Check sheet for the modelled part. Datum: model origin and axes. Units: mm. A direction names the side the tool comes from. Round coordinates to 2 decimals unless told otherwise and drop trailing zeros. Loops run counter-clockwise (first coordinate to the right, second up) from the corner with the lowest first, then second, coordinate; pieces in that order, holes last. Notation, with made-up numbers: M 38,68.5 L 80,68.5 A16 ccw 80,93.5 Z; hole C -9,-35 d3. An arc over 180 degrees is marked long. Write item = value, one per line. Start each with the question number.
(1) Scan lines: L1, parallel to Y at x = -0.05, z = 0.9; L2, parallel to X at y = 20, z = 1.6; L3, parallel to Y at x = -0.1, z = 0.45. Record each from-to range of solid material in increasing order. Write a range as from..to.
(2) Mould release check, pull along Y, two halves, no side actions. Record for faces 3 (the face through (-0.325, 21.464, 1.479)), 4 (the face through (1, 0, 0)): pulls with the +Y half, pulls with the -Y half, needs draft (parallel to the pull), parting line crosses it, or undercut.
(3) Cross-section at B-B on z = 0.25. Record the boundary of the cut face in (x, y).
(4) Cross-section at D-D on z = 1.9. Record the boundary of the cut face in (x, y).
(5) Cross-section at A-A on y = 20. Record the boundary of the cut face in (x, z).
(6) Cross-section at C-C on x = -0.2. Record the boundary of the cut face in (y, z), plus the area to 3 significant figures.
(7) Go/stop test with a flat-tipped pin: P1, Ø1, axis at y = 18, z = 2.5, coming from the -X side. Record where the tip stops, or that it passes through.
(8) Set-up check for faces 1 (the face through (-0.976, 9.876, 1.283)), 2 (the face through (-0.108, -0.488, 1.479)): record each of +Z, -Z, +X, -X, +Y, -Y from which the full face is reachable in a straight line by a thin tool's end or side.
from build123d import *

# Parameters (mm, degrees)
SKETCH_1_R           = 1.5
SKETCH_1_R_2         = 0.5
EXTRUDE_1_DEPTH      = 3
EXTRUDE_2_REACH      = 13.979
EXTRUDE_2_END_RADIUS = 1.5
SKETCH_2_R           = 1


with BuildPart() as part:
    # 草图1 → 凸台-拉伸1 (new body)
    with BuildSketch(Plane.XY):
        Circle(SKETCH_1_R)
        Circle(SKETCH_1_R_2, mode=Mode.SUBTRACT)
    extrude_1 = extrude(amount=EXTRUDE_1_DEPTH)

    # 凸台-拉伸2: up to this cylinder (the profile starts outside it)
    extrude_2_end = Plane(origin=(0, 0, 1.5), z_dir=(0, 0, -1)) * Cylinder(EXTRUDE_2_END_RADIUS, 31.958, mode=Mode.PRIVATE)
    # 草图2 → 凸台-拉伸2 (add, up to the surface)
    with BuildSketch(Plane(origin=(0, 10, 0), x_dir=(1, 0, 0), z_dir=(0, 1, 0)), mode=Mode.PRIVATE) as extrude_2_sk1:
        with Locations(Location((0, -1.5, 0), (0, 0, 270))):
            Circle(SKETCH_2_R)
    extrude_2_tool1 = extrude(extrude_2_sk1.sketch, amount=-EXTRUDE_2_REACH, mode=Mode.PRIVATE) - extrude_2_end
    extrude_2 = extrude_2_tool1.solids().sort_by_distance((0, 10, 1.5))[0]
    add(extrude_2)

    # 镜向1: 凸台-拉伸2 across plane
    add(extrude_2.mirror(Plane.ZX.offset(10)))

    # 镜向2: 凸台-拉伸1 across plane
    add(extrude_1.mirror(Plane.ZX.offset(10)))


solid = part.part
Result:
q1.L1 = -1.5..-0.5, 0.5..19.5, 20.5..21.5
q1.L2 = -1.5..-0.5, 0.5..1.5
q1.L3 = -1.5..-0.49, 0.49..1.5, 18.5..19.51, 20.49..21.5
q2.face_3 = undercut
q2.face_4 = needs draft
q3.outline = C 0,0 d3; C 0,20 d3; hole C 0,0 d1; hole C 0,20 d1
q4.outline = M -0.92,1.19 A1.5 ccw long 0.92,1.19 L 0.92,18.81 A1.5 ccw long -0.92,18.81 Z; hole C 0,0 d1; hole C 0,20 d1
q5.outline = M -1.5,0 L -0.5,0 L -0.5,3 L -1.5,3 Z; M 0.5,0 L 1.5,0 L 1.5,3 L 0.5,3 Z
q6.outline = M -1.49,0 L -0.46,0 L -0.46,3 L -1.49,3 Z; M 0.46,0 L 1.49,0 L 1.49,0.52 L 18.51,0.52 L 18.51,0 L 19.54,0 L 19.54,3 L 18.51,3 L 18.51,2.48 L 1.49,2.48 L 1.49,3 L 0.46,3 Z; M 20.46,0 L 21.49,0 L 21.49,3 L 20.46,3 Z
q6.area = 45.7 mm^2
q7.P1 = -0.87
q8.face_1 = none
q8.face_2 = +Z, -Z
